Design review of the part built by this model. Coordinates are the model's own, in mm. Coordinates: 2 decimals unless noted, no trailing zeros. Loops run counter-clockwise (first coordinate to the right, second up) from the corner with the lowest first, then second, coordinate; pieces in that order, holes last. Notation, with made-up numbers: (13.25, -3.5) -> (46.25, -3.5) arc R14 ccw to (46.25, 9.5) -> close; hole circle Ø9 at (10, 5.5). An arc over 180 degrees is marked (long way). Use one line per item in the form item = value. Start each with the question number.
1. Consider section A-A (x = 0). State the section outline as (y, z) points, then the cut area to 3 significant figures.
2. Wall thickness on line 1 (Z direction, x = 0.5, y = 41); line 2 (X direction, y = 15, z = 5.5); line 3 (Z direction, x = -12.5, y = 45.5): over which ranges is each line inside the solid? List them lowest first. Write a range as from..to.
3. Consider section B-B (z = 0). State the section outline as (x, y) points.
4. For pin 1 (4 mm diameter, centred on x = 14, z = -6, fed in from -Y); pin 2 (1 mm diameter, centred on x = 12, y = 42.5, fed in from +Z); pin 3 (6 mm diameter, centred on y = 89.5, z = 13.5, fed in from -X), all flat-tipped, find the tip position at first contact; note any pin that passes through.
5. Consider section D-D (y = 12). State the section outline as (x, z) points, then the cut area to 3 significant figures.
6. Consider section C-C (y = 91.5). State the section outline as (x, z) points.
from build123d import *

# Parameters (mm, degrees)
SKETCH2_R               = 19.05
BOSS_EXTRUDE1_DEPTH     = 114.3
CUT_EXTRUDE5_DEPTH      = 20.05
CUT_EXTRUDE5_DEPTH_BACK = 20.05


with BuildPart() as part:
    # Sketch1 → Revolve1 (revolve)
    with BuildSketch(Plane.XY):
        Polygon((0, 26.065803987), (19.05, 26.065803987), (0, -12.034196013), align=None)
    revolve(axis=Axis((0, 32.664443941, 0), (0, -1, 0)))

    # Sketch2 → Boss-Extrude1 (add)
    with BuildSketch(Plane(origin=(0, 26.065803987, 0), x_dir=(1, 0, 0), z_dir=(0, 1, 0))):
        Circle(SKETCH2_R)
    extrude(amount=BOSS_EXTRUDE1_DEPTH)

    # Sketch4 → Cut-Extrude5 (cut, two sides)
    with BuildSketch(Plane.XY) as cut_extrude5_sk:
        Polygon((-7.278791919, 2.523387825), (7.278791919, 2.523387825), (0, -12.034196013), align=None)
    extrude(amount=CUT_EXTRUDE5_DEPTH, mode=Mode.SUBTRACT)
    extrude(cut_extrude5_sk.sketch, amount=-CUT_EXTRUDE5_DEPTH_BACK, mode=Mode.SUBTRACT)


solid = part.part
Geometry check:
q1.outline = (2.52, -7.28) -> (26.07, -19.05) -> (140.37, -19.05) -> (140.37, 19.05) -> (26.07, 19.05) -> (2.52, 7.28) -> close
q1.area = 4,970 mm²
q2.line_1 = -19.04..19.04
q2.line_2 = -12.35..12.35
q2.line_3 = -14.38..14.38
q3.outline = (-19.05, 26.07) -> (-7.28, 2.52) -> (7.28, 2.52) -> (19.05, 26.07) -> (19.05, 140.37) -> (-19.05, 140.37) -> close
q4.pin_1 = 14.43
q4.pin_2 = 15.19
q4.pin_3 = -15.9
q5.outline = circle Ø24.03 at (0, 0)
q5.area = 454 mm²
q6.outline = circle Ø38.1 at (0, 0)
